Check sheet for the drawn part. Datum: minimum x, y, z corner. Units: mm. Round coordinates to 2 decimals unless told otherwise and drop trailing zeros. Write each loop counter-clockwise with the first axis right and the second up, starting at its lowest first coordinate (ties: lowest second). Pieces come first, ordered by that corner, then holes. Notation, with made-up numbers: (67, 35) -> (82, 35) arc R20 cw to (82, 74) -> close; hole circle Ø2 at (33.25, -23). An arc over 180 degrees is marked (long way). Use CSV: the item, a comma, the result in double quotes.
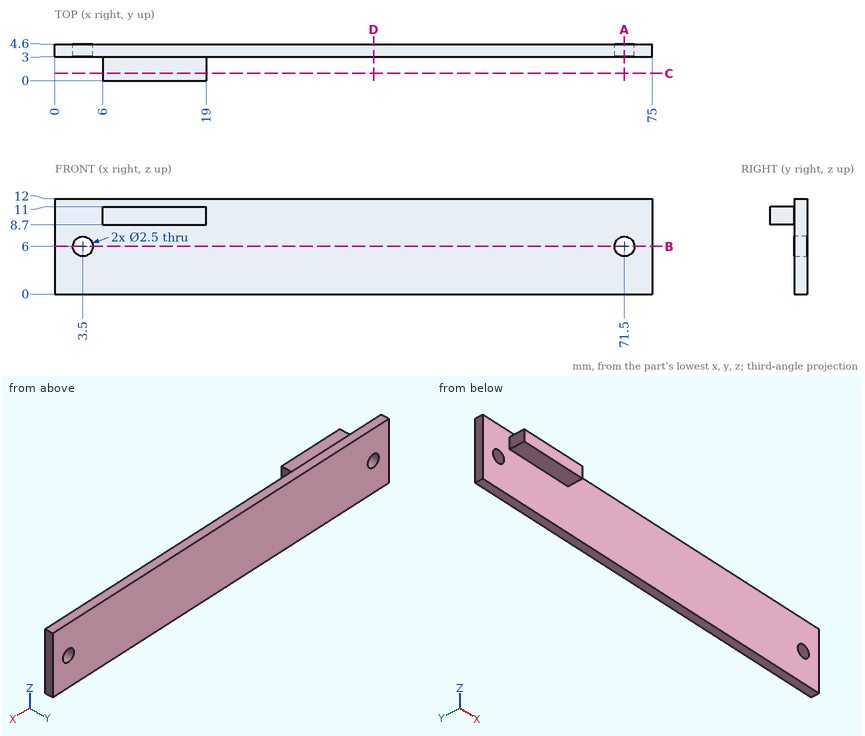
Q1. Section check A-A (x = 71.5). Record the cut outline in (y, z).
Filled in:
outline,"(3, 0) -> (4.6, 0) -> (4.6, 4.75) -> (3, 4.75) -> close; (3, 7.25) -> (4.6, 7.25) -> (4.6, 12) -> (3, 12) -> close"
Q2. Section check D-D (x = 40). Record the cut outline in (y, z).
Filled in:
outline,"(3, 0) -> (4.6, 0) -> (4.6, 12) -> (3, 12) -> close"
Q3. Section check B-B (z = 6). Record the cut outline in (x, y), plus the area to 3 significant figures.
Filled in:
outline,"(0, 3) -> (2.25, 3) -> (2.25, 4.6) -> (0, 4.6) -> close; (4.75, 3) -> (70.25, 3) -> (70.25, 4.6) -> (4.75, 4.6) -> close; (72.75, 3) -> (75, 3) -> (75, 4.6) -> (72.75, 4.6) -> close"
area,"112 mm²"
Q4. Material ranges on L1, parallel to X at y = 3.85, z = 6; L2, parallel to Z at x = 3.5, y = 3.4; L3, parallel to Y at x = 46.5, z = 4.5, recorded low to high.
Filled in:
L1,"0 to 2.25, 4.75 to 70.25, 72.75 to 75"
L2,"0 to 4.75, 7.25 to 12"
L3,"3 to 4.6"
Q5. Section check C-C (y = 0.9). Record the cut outline in (x, z).
Filled in:
outline,"(6, 8.7) -> (19, 8.7) -> (19, 11) -> (6, 11) -> close"
Q6. Go/stop test with flat-tipped pins: P1, Ø6, axis at x = 13.5, z = 5.5, coming from the -Y side; P2, Ø1.2, axis at y = 2, z = 9.5, coming from the +X side; P3, Ø2.5, axis at x = 9.5, y = 1.5, coming from the -Z side. Record where each tip stops, or that it passes through.
Filled in:
P1,"y = 3"
P2,"x = 19"
P3,"z = 8.7"
